Autodesk Inventor part; units mm, degrees
ref_plane "Pracovní rovina2" through (0, 0, 3) normal (0, 0, 1) x (1, 0, 0)
ref_plane "YZ Plane" through (0, 0, 0) normal (1, 0, 0) x (0, 1, 0)
ref_plane "XZ Plane" through (0, 0, 0) normal (0, 1, 0) x (-1, 0, 0)
sketch "Náčrt1" plane through (0, 0, 0) normal (0, 0, 1) x (1, 0, 0)
  line L0 (0, 35) -> (0, -35)
  line L1 (-29.75, 0) -> (29.75, 0)
  line L2 (21.25, -25) -> (-21.25, -25)
  line L3 (-21.25, -25) -> (-21.25, 25)
  line L4 (-21.25, 25) -> (21.25, 25)
  line L5 (21.25, 25) -> (21.25, -25)
  point P0 (0, 0)
  dimension "d0" = 42.5
  dimension "d1" = 50
extrude "Vysunutí1" add sketch "Náčrt1" along normal blind 3
sketch "Náčrt2" plane through (0, 0, 3) normal (0, 0, 1) x (1, 0, 0)
  line L0 (21.25, 25) -> (-21.25, 25)
  line L1 (-21.25, 25) -> (-21.25, -25)
  line L2 (-21.25, -25) -> (21.25, -25)
  line L3 (21.25, -25) -> (21.25, 25)
  line L4 (0, 35) -> (0, -35)
  line L5 (-29.75, 0) -> (29.75, 0)
  line L6 (4.5, -18.5) -> (-3.5, -18.5)
  line L7 (-3.5, -18.5) -> (-3.5, -15.5)
  line L8 (-3.5, -15.5) -> (4.5, -15.5)
  line L9 (4.5, -15.5) -> (4.5, -18.5)
  line L10 (14.5, -17.5) -> (11.5, -17.5)
  line L11 (11.5, -17.5) -> (11.5, -5.5)
  line L12 (11.5, -5.5) -> (14.5, -5.5)
  line L13 (14.5, -5.5) -> (14.5, -17.5)
  line L14 (-17.5, 21.5) -> (17.5, 21.5) construction
  line L15 (17.5, 21.5) -> (17.5, -21.5) construction
  line L16 (17.5, -21.5) -> (-17.5, -21.5) construction
  line L17 (-17.5, -21.5) -> (-17.5, 21.5) construction
  point P0 (0, 0)
  dimension "d4" = 12
  dimension "d5" = 3
  dimension "d6" = 8
  dimension "d7" = 3
  dimension "d9" = 35
  dimension "d10" = 43
  dimension "d11" = 3
  dimension "d13" = 3
  dimension "d29" = 16
  dimension "d30" = 21
extrude "Vysunutí2" cut sketch "Náčrt2" against normal through all contours L8 L9 L6 L4 | L4 L6 L7 L8 | L10 L11 L12 L13
sketch "Náčrt3" plane through (0, 0, 3) normal (0, 0, 1) x (1, 0, 0)
  line L0 (-3.5, -18.5) -> (-3.5, -15.5)
  line L1 (-3.5, -15.5) -> (4.5, -15.5)
  line L2 (4.5, -15.5) -> (4.5, -18.5)
  line L3 (4.5, -18.5) -> (-3.5, -18.5)
  line L4 (11.5, -17.5) -> (11.5, -5.5)
  line L5 (11.5, -5.5) -> (14.5, -5.5)
  line L6 (14.5, -5.5) -> (14.5, -17.5)
  line L7 (14.5, -17.5) -> (11.5, -17.5)
  line L8 (21.25, 25) -> (-21.25, 25)
  line L9 (-21.25, 25) -> (-21.25, -25)
  line L10 (-21.25, -25) -> (21.25, -25)
  line L11 (21.25, -25) -> (21.25, 25)
  line L12 (0, 38.5) -> (0, -38.5)
  line L13 (-33.25, 0) -> (33.25, 0)
  line L14 (-19, 22.75) -> (19, 22.75)
  line L15 (19, 22.75) -> (19, -22.75)
  line L16 (19, -22.75) -> (-19, -22.75)
  line L17 (-19, -22.75) -> (-19, 22.75)
  line L18 (-21, 24.75) -> (21, 24.75)
  line L19 (21, 24.75) -> (21, -24.75)
  line L20 (21, -24.75) -> (-21, -24.75)
  line L21 (-21, -24.75) -> (-21, 24.75)
  point P0 (0, 0)
  dimension "d31" = 0.25
  dimension "d32" = 2
extrude "Vysunutí3" add sketch "Náčrt3" along normal blind 3 contours L16 L15 L13 L19 L20 L12 | L12 L20 L21 L13 L17 L16 | L14 L17 L13 L21 L18 L12 | L12 L18 L19 L13 L15 L14
sketch "Náčrt6" plane through (0, 0, 0) normal (0, 0, -1) x (-1, 0, 0)
  line L0 (3.5, -15.5) -> (3.5, -18.5)
  line L1 (3.5, -18.5) -> (-4.5, -18.5)
  line L2 (-4.5, -18.5) -> (-4.5, -15.5)
  line L3 (-4.5, -15.5) -> (3.5, -15.5)
  line L4 (-11.5, -5.5) -> (-11.5, -17.5)
  line L5 (-11.5, -17.5) -> (-14.5, -17.5)
  line L6 (-14.5, -17.5) -> (-14.5, -5.5)
  line L7 (-14.5, -5.5) -> (-11.5, -5.5)
  line L8 (-21.25, 25) -> (21.25, 25)
  line L9 (-21.25, -25) -> (-21.25, 25)
  line L10 (21.25, -25) -> (-21.25, -25)
  line L11 (21.25, 25) -> (21.25, -25)
  line L12 (0, -35) -> (0, 35)
  line L13 (-29.75, 0) -> (29.75, 0)
  line L14 (23.75, 27.5) -> (-23.75, 27.5)
  line L15 (-23.75, 27.5) -> (-23.75, -27.5)
  line L16 (-23.75, -27.5) -> (23.75, -27.5)
  line L17 (23.75, -27.5) -> (23.75, 27.5)
  point P0 (0, 0)
  dimension "d33" = 2.5
extrude "Vysunutí6" add sketch "Náčrt6" against normal up to surface (3 mm away) contours L12 L16 L15 L13 L9 L10 | L10 L11 L13 L17 L16 L12 | L12 L14 L17 L13 L11 L8 | L8 L9 L13 L15 L14 L12
ref_plane "Pracovní rovina1" through (0, 0, 1.5) normal (0, 0, -1) x (-1, 0, 0)
mirror "Zrcadlit1" about plane through (0, 0, 1.5) normal (0, 0, -1) of "Vysunutí3"
ref_plane "Pracovní rovina2" through (0, 0, 3) normal (0, 0, 1) x (1, 0, 0)
split "Rozdělit1" plane through (0, 0, 3) removes the side toward (0, 0, 1)
fillet "Zaoblení4" radius 2 8 edges at (23.75, 27.5, 1.5) (23.75, 0, 3) (0, 27.5, 3) (23.75, -27.5, 1.5) (0, -27.5, 3) (-23.75, 27.5, 1.5) (-23.75, 0, 3) (-23.75, -27.5, 1.5)
properties part number "a4988_box_lid_3D tisk"
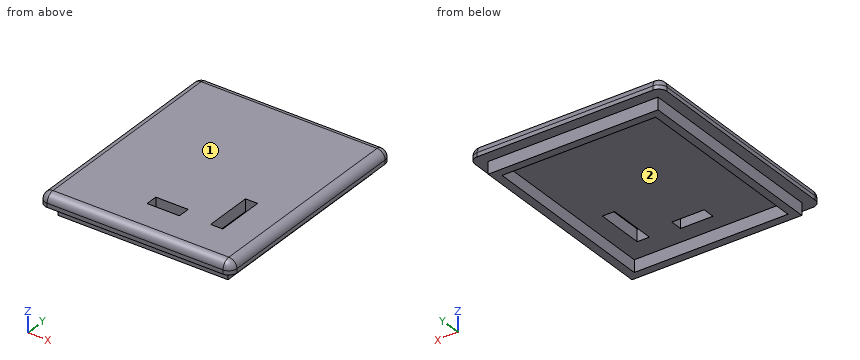
Can you work these out from the model? Positions are in its coordinate system, mm. Face numbers are marked on the shaded views. Coordinates: 2 decimals unless noted, no trailing zeros. Write each loop counter-clockwise with the first axis right and the second up, starting at its lowest first coordinate (ties: lowest second). Pieces come first, ordered by that corner, then holes. Notation, with made-up numbers: (38, 26) - (68, 26) arc R22 ccw to (68, 57) - close; hole circle Ø7 at (-36.75, 23.5). An arc over 180 degrees is marked (long way). Return JSON: item names as keys, results as strings. Group by question number.
Item 1: If we section it at A-A (x = 1): Write out the boundary of the cut face in (y, z), then the cut area to 3 significant figures.
Item 2: If we section it at D-D (x = -7): Write out the boundary of the cut face in (y, z).
Item 3: I'm going to push flat-ended pins straight in: pin 1 Ø1.5 at (x, y) = (-9, 0.5) entering from -Z; pin 2 Ø1.5 at (x, z) = (3, -1.5) entering from +Y; pin 3 Ø0.9 at (x, z) = (4, -1) entering from -Y. Where does each tip first touch, or does it pass through?
Item 4: If we section it at B-B (z = 2.2): Write out the boundary of the cut face in (x, y), then the cut area to 3 significant figures.
Item 5: We'd pull the mould along Y, two halves only. Please class the marked faces 1 and 2: pulls with the +Y half, pulls with the -Y half, needs draft (parallel to the pull), parting line crosses it, or undercut.
Item 6: Please list where these lines run through material, in increasing order: probe 1 along X at (y, z) = (-11, 0.5); probe 2 along Y at (x, z) = (-17.5, -1.9); probe 3 along X at (y, z) = (19.5, -2).
Item 7: If we section it at C-C (y = -8.5): Write out the boundary of the cut face in (x, z).
Return value:
{
 "1": {"outline": "(-27.5, 0) - (-24.75, 0) - (-24.75, -3) - (-22.75, -3) - (-22.75, 0) - (-18.5, 0) - (-18.5, 3) - (-25.5, 3) arc R2 ccw to (-27.5, 1) - close; (-15.5, 0) - (22.75, 0) - (22.75, -3) - (24.75, -3) - (24.75, 0) - (27.5, 0) - (27.5, 1) arc R2 ccw to (25.5, 3) - (-15.5, 3) - close", "area": "166 mm^2"},
 "2": {"outline": "(-27.5, 0) - (-24.75, 0) - (-24.75, -3) - (-22.75, -3) - (-22.75, 0) - (22.75, 0) - (22.75, -3) - (24.75, -3) - (24.75, 0) - (27.5, 0) - (27.5, 1) arc R2 ccw to (25.5, 3) - (-25.5, 3) arc R2 ccw to (-27.5, 1) - close"},
 "3": {"pin 1": "stops at z = 0", "pin 2": "stops at y = 24.75", "pin 3": "stops at y = -24.75"},
 "4": {"outline": "(-23.35, -25.5) arc R1.6 ccw to (-21.75, -27.1) - (21.75, -27.1) arc R1.6 ccw to (23.35, -25.5) - (23.35, 25.5) arc R1.6 ccw to (21.75, 27.1) - (-21.75, 27.1) arc R1.6 ccw to (-23.35, 25.5) - close; hole (-3.5, -18.5) - (4.5, -18.5) - (4.5, -15.5) - (-3.5, -15.5) - close; hole (11.5, -17.5) - (14.5, -17.5) - (14.5, -5.5) - (11.5, -5.5) - close", "area": "2,470 mm^2"},
 "5": {"face 1": "needs draft", "face 2": "undercut"},
 "6": {"probe 1": "x = -23.75 to 11.5, 14.5 to 23.75", "probe 2": "y = -24.75 to -22.75, 22.75 to 24.75", "probe 3": "x = -21 to -19, 19 to 21"},
 "7": {"outline": "(-23.75, 0) - (-21, 0) - (-21, -3) - (-19, -3) - (-19, 0) - (11.5, 0) - (11.5, 3) - (-21.75, 3) arc R2 ccw to (-23.75, 1) - close; (14.5, 0) - (19, 0) - (19, -3) - (21, -3) - (21, 0) - (23.75, 0) - (23.75, 1) arc R2 ccw to (21.75, 3) - (14.5, 3) - close"}
}
